from build123d import *

# Parameters (mm, degrees)
F0_W     = 41.662812
F0_H     = 20
F0_R     = 11.641019
F0_R_2   = 7.924866
F0_R_3   = 7.996653
F1_DEPTH = 25
F2_DEPTH = 25


with BuildPart() as f1:
    # F0 (on Front) → F1 (new body)
    with BuildSketch(Plane.XZ):
        Polygon((-73.644338, 49.131665), (-98.355876, 49.131665), (-98.355876, -50.868335), (-56.336644, -50.868335), (-48.355876, -61.926026), (-48.355876, -71.541415), (71.644124, -71.541415), (71.644124, -50.868335), (101.644124, -50.868335), (101.644124, 49.131665), (71.644124, 49.131665), (71.644124, 89.131665), (-68.355876, 89.131665), (-68.355876, 64.035509), align=None)
        Polygon((-88.355876, -45.193389), (-88.355876, -25.193389), (-62.702298, -25.193389), (-62.702298, -38.416974), (-68.994693, -45.193389), align=None, mode=Mode.SUBTRACT)
        with Locations((-67.52447, -10)):
            Rectangle(F0_W, F0_H, mode=Mode.SUBTRACT)
        with Locations((76.690935, -27.195666)):
            Circle(F0_R, mode=Mode.SUBTRACT)
        with Locations((79.56899, 0)):
            Circle(F0_R_2, mode=Mode.SUBTRACT)
        Polygon((-88.355876, 20.634644), (-88.355876, 36.607623), (-68.38667, 37.717025), (-61.126228, 29.488518), (-61.126228, 20.634644), align=None, mode=Mode.SUBTRACT)
        Polygon((-33.624265, 50.160453), (-26.363822, 59.841048), (35.10794, 59.841048), (43.820471, 48.224337), (43.820471, -33.576678), (46.346532, -39.643808), (-33.624265, -41.805182), align=None, mode=Mode.SUBTRACT)
        with Locations((75.539708, 26.911816)):
            Circle(F0_R_3, mode=Mode.SUBTRACT)
    extrude(amount=F1_DEPTH)

    # F0 (on Front) → F2 (join)
    with BuildSketch(Plane.XZ):
        Polygon((-73.644338, 49.131665), (-98.355876, 49.131665), (-98.355876, -50.868335), (-56.336644, -50.868335), (-48.355876, -61.926026), (-48.355876, -71.541415), (71.644124, -71.541415), (71.644124, -50.868335), (101.644124, -50.868335), (101.644124, 49.131665), (71.644124, 49.131665), (71.644124, 89.131665), (-68.355876, 89.131665), (-68.355876, 64.035509), align=None)
        Polygon((-88.355876, -45.193389), (-88.355876, -25.193389), (-62.702298, -25.193389), (-62.702298, -38.416974), (-68.994693, -45.193389), align=None, mode=Mode.SUBTRACT)
        with Locations((-67.52447, -10)):
            Rectangle(F0_W, F0_H, mode=Mode.SUBTRACT)
        with Locations((76.690935, -27.195666)):
            Circle(F0_R, mode=Mode.SUBTRACT)
        with Locations((79.56899, 0)):
            Circle(F0_R_2, mode=Mode.SUBTRACT)
        Polygon((-88.355876, 20.634644), (-88.355876, 36.607623), (-68.38667, 37.717025), (-61.126228, 29.488518), (-61.126228, 20.634644), align=None, mode=Mode.SUBTRACT)
        Polygon((-33.624265, 50.160453), (-26.363822, 59.841048), (35.10794, 59.841048), (43.820471, 48.224337), (43.820471, -33.576678), (46.346532, -39.643808), (-33.624265, -41.805182), align=None, mode=Mode.SUBTRACT)
        with Locations((75.539708, 26.911816)):
            Circle(F0_R_3, mode=Mode.SUBTRACT)
    extrude(amount=F2_DEPTH)


solid = f1.part
CAD build for the part. Positions are in the model's coordinates, mm. A direction names the side the tool comes from. Round coordinates to 2 decimals unless told otherwise and drop trailing zeros. Order: outer loops, then holes, each group sorted by start corner. A loop starts at its lowest first (then second) coordinate and runs counter-clockwise, first axis right, second up. Notation, with made-up numbers: (41.5, 41.5) - (77.5, 41.5) arc R10 cw to (77.5, 48.5) - close; hole circle Ø7 at (16, 38.5). An arc over 180 degrees is marked (long way). Return JSON: item names as keys, results as strings.
(1) Cut at A-A (z = -10). Give the cut face in (x, y), then the cut area to 3 significant figures.
Answer key:
{"outline": "(-98.36, -25) - (-88.36, -25) - (-88.36, 0) - (-98.36, 0) - close; (-46.69, -25) - (-33.62, -25) - (-33.62, 0) - (-46.69, 0) - close; (43.82, -25) - (101.64, -25) - (101.64, 0) - (43.82, 0) - close", "area": "2,020 mm^2"}
(2) Pin check, flat tips, straight feed: pin 1 Ø7.5 at (x, y) = (-91, -8) entering from +Z; pin 2 Ø12.5 at (x, y) = (-77, -7.5) entering from -Z; pin 3 Ø12 at (x, z) = (35.5, 35.5) entering from +Y. Stop position of each tip, or through.
Answer key:
{"pin 1": "stops at z = 49.13", "pin 2": "stops at z = -50.87", "pin 3": "passes through"}
(3) Wall check: probe 1 along X at (y, z) = (-15, 27.5); probe 2 along X at (y, z) = (-14.5, -13.5); probe 3 along X at (y, z) = (-10.25, 44.5). Give the ranges that are in metal, low to high. Write a range as from..to.
Answer key:
{"probe 1": "x = -98.36..-88.36, -61.13..-33.62, 43.82..67.56, 83.51..101.64", "probe 2": "x = -98.36..-88.36, -46.69..-33.62, 43.82..101.64", "probe 3": "x = -98.36..-33.62, 43.82..101.64"}
(4) Pull direction Z, two halves, no side cores. Call faces 5 (the face through (43.82, -12, 8)), 6 (the face through (-88.356, -12, 29)), 7 (the face through (11, -12, -71.541)), 8 (the face through (-86, -12, 49.132)): +Z half, -Z half, draft (parallel to the pull), parting line (faces both ways), or undercut.
Answer key:
{"face 5": "undercut", "face 6": "undercut", "face 7": "-Z half", "face 8": "+Z half"}
(5) Cut at C-C (z = 32). Give the cut face in (x, y).
Answer key:
{"outline": "(-98.36, -25) - (-88.36, -25) - (-88.36, 0) - (-98.36, 0) - close; (-63.34, -25) - (-33.62, -25) - (-33.62, 0) - (-63.34, 0) - close; (43.82, -25) - (69.37, -25) - (69.37, 0) - (43.82, 0) - close; (81.71, -25) - (101.64, -25) - (101.64, 0) - (81.71, 0) - close"}
(6) Tool access for faces 1 (the face through (45, -25, 10)), 2 (the face through (-78, -12, -50.868)), 3 (the face through (71.644, -12, -61)), 4 (the face through (-64.807, -12.325, 33.66)): list every direction of +Z, -Z, +X, -X, +Y, -Y with a clear straight run to the whole face (end or side of a thin tool).
Answer key:
{"face 1": "+Z, -Z, +X, -X, -Y", "face 2": "-Z, -X, +Y, -Y", "face 3": "-Z, +X, +Y, -Y", "face 4": "+Y, -Y"}
(7) Cut at D-D (x = 11). Give the cut face in (y, z), then the cut area to 3 significant figures.
Answer key:
{"outline": "(-25, -71.54) - (0, -71.54) - (0, -40.6) - (-25, -40.6) - close; (-25, 59.84) - (0, 59.84) - (0, 89.13) - (-25, 89.13) - close", "area": "1,510 mm^2"}
(8) Cut at B-B (x = -65.5). Give the cut face in (y, z).
Answer key:
{"outline": "(-25, -50.87) - (0, -50.87) - (0, -41.43) - (-25, -41.43) - close; (-25, -25.19) - (0, -25.19) - (0, -20) - (-25, -20) - close; (-25, 0) - (0, 0) - (0, 20.63) - (-25, 20.63) - close; (-25, 34.45) - (0, 34.45) - (0, 89.13) - (-25, 89.13) - close"}
